Autodesk Inventor part; units mm, degrees
ref_plane "YZ Plane" through (0, 0, 0) normal (1, 0, 0) x (0, 1, 0)
ref_plane "XZ Plane" through (0, 0, 0) normal (0, 1, 0) x (-1, 0, 0)
ref_plane "XY Plane" through (0, 0, 0) normal (0, 0, 1) x (1, 0, 0)
sketch "Sketch1" plane through (0, 0, 0) normal (0, 0, 1) x (1, 0, 0)
  line L0 (0, 0) -> (50.8, 0)
  line L1 (50.8, 0) -> (50.8, 25.4)
  line L2 (50.8, 25.4) -> (0, 25.4)
  line L3 (0, 25.4) -> (0, 0)
  dimension "d0" = 50.8
  dimension "d1" = 25.4
extrude "Extrusion1" add sketch "Sketch1" along normal blind 38.1
sketch "Sketch2" plane through (0, 0, 38.1) normal (0, 0, 1) x (1, 0, 0)
  line L0 (0, 0) -> (50.8, 0)
  line L1 (50.8, 0) -> (50.8, 25.4)
  line L2 (50.8, 25.4) -> (0, 25.4)
  line L3 (0, 25.4) -> (0, 0)
  line L4 (6.35, 25.4) -> (44.45, 25.4)
  line L5 (44.45, 25.4) -> (44.45, 6.35)
  line L6 (44.45, 6.35) -> (6.35, 6.35)
  line L7 (6.35, 6.35) -> (6.35, 25.4)
  dimension "d4" = 6.35
  dimension "d5" = 6.35
  dimension "d6" = 6.35
extrude "Extrusion2" cut sketch "Sketch2" against normal through all contours L2 L5 L6 L7
equation "\"d5\" = d4"
equation "\"d6\" = d4"
properties part number "To Next Termination"
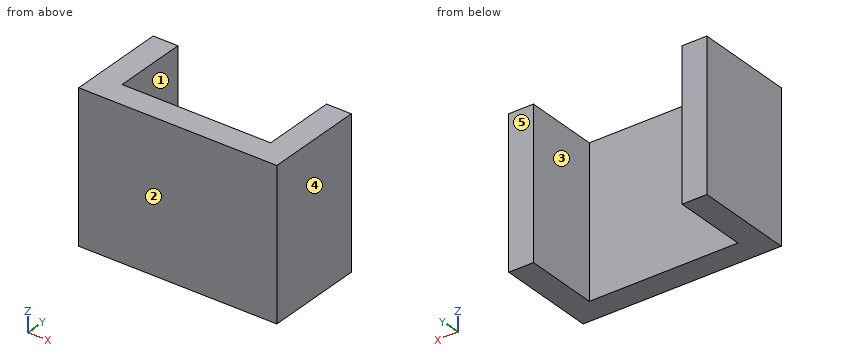
Work out the finished part from the listing and answer in its coordinate system (mm). Face numbers are marked on the shaded views. A direction names the side the tool comes from. Give positions to 0.01 mm unless a question says otherwise; leave off trailing zeros. Write each loop counter-clockwise with the first axis right and the second up, starting at its lowest first coordinate (ties: lowest second). Pieces come first, ordered by that corner, then holes. Notation, with made-up numbers: (-34, -36.75) -> (-20, -36.75) arc R15 ccw to (-20, -26.75) -> close; hole circle Ø5 at (49, 67.5). An arc over 180 degrees is marked (long way). Write item = value, one per line.
Q1. Section C-C on x = 13 is taken. Determine the outline of the cut face in (y, z).
Computed values:
outline = (0, 0) -> (6.35, 0) -> (6.35, 38.1) -> (0, 38.1) -> close
Q2. A tool of negligible diameter and unlimited length cuts with its end or side. For the marked faces 1 and 2, from which of +Z, -Z, +X, -X, +Y, -Y can it reach the whole face along a straight path? Write none if from no direction.
Computed values:
face_1 = +Z, -Z, +Y
face_2 = +Z, -Z, +X, -X, -Y
Q3. Section A-A on y = 16 is taken. Determine the outline of the cut face in (x, z).
Computed values:
outline = (0, 0) -> (6.35, 0) -> (6.35, 38.1) -> (0, 38.1) -> close; (44.45, 0) -> (50.8, 0) -> (50.8, 38.1) -> (44.45, 38.1) -> close
Q4. Consider line 1 along X through (y, z) = (7, 26.5); line 2 along Y through (x, z) = (43, 6). Determine where each line is inside the solid, lowest interval first.
Computed values:
line_1 = 0 to 6.35, 44.45 to 50.8
line_2 = 0 to 6.35
Q5. A flat-ended cylindrical pin translates along its axis: pin 1 Ø2 at (x, z) = (36, 12.5) entering from +Y. Find the tip coordinate at first contact, or state that the pin passes through.
Computed values:
pin_1 = 6.35
Q6. Section B-B on z = 24 is taken. Determine the outline of the cut face in (x, y), and give its area (3 significant figures).
Computed values:
outline = (0, 0) -> (50.8, 0) -> (50.8, 25.4) -> (44.45, 25.4) -> (44.45, 6.35) -> (6.35, 6.35) -> (6.35, 25.4) -> (0, 25.4) -> close
area = 565 mm^2
Q7. For a pull along X with two mould halves and no side action, classify the marked faces 3, 4 and 5 as pulls with the +X half, pulls with the -X half, needs draft (parallel to the pull), parting line crosses it, or undercut.
Computed values:
face_3 = undercut
face_4 = pulls with the +X half
face_5 = needs draft
